Can you work these out from the model? Positions are in its coordinate system, mm. Coordinates: 2 decimals unless noted, no trailing zeros. Order: outer loops, then holes, each group sorted by start corner. A loop starts at its lowest first (then second) coordinate and runs counter-clockwise, first axis right, second up. Notation, with made-up numbers: M -29.5,-27 L 29.5,-27 A22 cw 29.5,9 Z; hole C 14,65.5 d3. An arc over 180 degrees is marked long. Answer as CSV lines item,"result". Start each with the question number.
1. I need wall thicknesses on line 1 along Y through (x, z) = (218, 2.5); line 2 along Y through (x, z) = (196.85, 1.2); line 3 along Y through (x, z) = (66.5, 3.2). Which ranges of each line are inside material? Lowest first, please. Write a range as from..to.
2. Will this pin go through, and if not, where does the flat tip stop? pin 1 (3 mm diameter, centred on x = 424, z = 3.5, fed in from +Y).
3. If we section it at A-A (x = 50.8): List the corners of the cut face in (y, z) for me, plus the area to 3 significant figures.
4. If we section it at B-B (z = 3.1): Give the number of separate pieces and of enclosed holes in the cut face, plus the area to 3 significant figures.
5. If we section it at C-C (y = 230): List the corners of the cut face in (x, z) for me, plus the area to 3 significant figures.
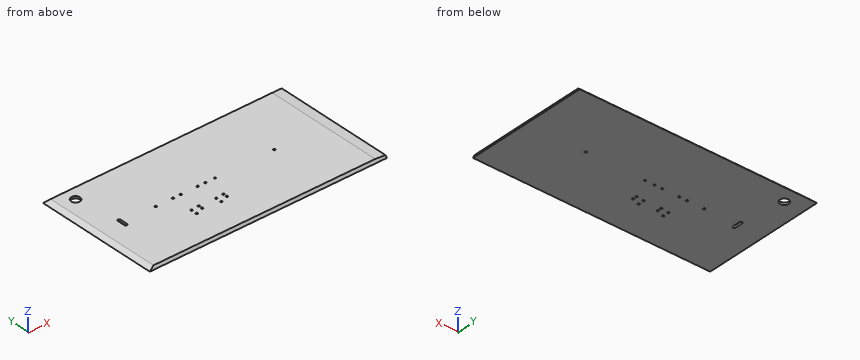
Autodesk Inventor part; units mm, degrees
ref_plane "YZ Plane" through (0, 0, 0) normal (1, 0, 0) x (0, 1, 0)
ref_plane "XY Plane" through (0, 0, 0) normal (0, 0, 1) x (1, 0, 0)
sketch "Sketch1" plane through (0, 0, 0) normal (0, 0, 1) x (1, 0, 0)
  line L0 (0, 0) -> (609.6, 0)
  line L1 (609.6, 0) -> (609.6, 317.881)
  line L2 (609.6, 317.881) -> (0, 317.881)
  line L3 (0, 317.881) -> (0, 0)
  dimension "d0" = 609.6
  dimension "d1" = 317.881
extrude "Extrusion1" add sketch "Sketch1" along normal blind 5.7658
sketch "Sketch2" plane through (0, 317.881, 0) normal (0, 1, 0) x (1, 0, 0)
  line L0 (609.6, 0) -> (0, 0)
  line L1 (0, 0) -> (0, -5.7658)
  line L2 (609.6, -5.7658) -> (0, -5.7658)
  line L3 (609.6, 0) -> (609.6, -5.7658)
  line L4 (0, 0) -> (609.6, 0)
  line L5 (0, 0) -> (14.4594, -5.7658)
  line L6 (0, -5.7658) -> (609.6, -5.7658)
  line L7 (14.4594, -5.7658) -> (14.4594, 0)
  line L8 (14.4594, -5.7658) -> (20.2252, -5.7658) construction
  dimension "d4" = 21.74
  dimension "d5" = 90
extrude "Extrusion2" cut sketch "Sketch2" against normal through all contours L5 L2 L1
sketch "Sketch3" plane through (609.6, 0, 0) normal (1, 0, 0) x (0, 0, -1)
  line L0 (0, 0) -> (0, 317.881)
  line L1 (0, 317.881) -> (-5.7658, 317.881)
  line L2 (-5.7658, 0) -> (-5.7658, 317.881)
  line L3 (0, 0) -> (-5.7658, 0)
  line L4 (0, 0) -> (-5.7658, 0)
  line L5 (0, 0) -> (-5.7658, 5.7658)
  line L6 (-5.7658, 0) -> (-5.7658, 317.881)
  line L7 (0, 0) -> (8.1541, 0) construction
  line L8 (0, 317.881) -> (-5.7658, 317.881)
  line L9 (0, 317.881) -> (-5.7658, 312.1152)
  line L10 (0, 317.881) -> (8.1541, 317.881) construction
  dimension "d8" = 135
  dimension "d9" = 135
extrude "Extrusion3" cut sketch "Sketch3" against normal through all contours L3 L2 L5 | L9 L2 L1
ref_plane "Center Plane" through (0, 158.9405, 0) normal (0, 1, 0) x (-1, 0, 0)
sketch "Sketch4" plane through (0, 158.9405, 0) normal (0, 1, 0) x (-1, 0, 0)
  line L0 (-14.4594, 5.7658) -> (0, 0)
  line L1 (-609.6, 5.7658) -> (-14.4594, 5.7658)
  line L2 (-609.6, 0) -> (-609.6, 5.7658)
  line L3 (-609.6, 0) -> (0, 0)
  line L4 (-609.6, 5.7658) -> (-584.2, 5.7658) construction
  line L5 (-584.2, 5.7658) -> (-609.6, 4.4413)
  point P0 (0, 0)
  dimension "d13" = 25.4
  dimension "d14" = 2.985
extrude "Extrusion4" cut sketch "Sketch4" against normal through all both and the other way through all contours L5 L2 L1
sketch "Sketch5" plane through (0, 0, 5.7658) normal (0, 0, 1) x (1, 0, 0)
  circle A0 centre (196.85, 158.9278) radius 2.5019
  line L0 (0, 317.881) -> (0, 0)
  line L1 (609.6, 317.881) -> (0, 317.881)
  circle A1 centre (260.35, 158.9405) radius 2.5019
  circle A2 centre (196.85, 103.5558) radius 2.5019
  circle A3 centre (260.35, 103.5685) radius 2.5019
  circle A4 centre (196.85, 88.3158) radius 2.5019
  circle A5 centre (260.35, 88.3285) radius 2.5019
  circle A6 centre (152.4, 158.9405) radius 2.5019
  circle A7 centre (304.8, 158.9405) radius 2.5019
  circle A8 centre (457.2, 158.9405) radius 2.5019
  line L2 (66.675, 145.7528) -> (67.325, 145.7528)
  line L3 (70.5, 148.9278) -> (70.5, 168.9278)
  line L4 (67.325, 172.1028) -> (66.675, 172.1028)
  line L5 (63.5, 168.9278) -> (63.5, 148.9278)
  line L6 (63.5, 145.7528) -> (70.5, 172.1028) construction
  line L7 (70.5, 145.7528) -> (63.5, 172.1028) construction
  arc A9 (70.5, 168.9278) -> (67.325, 172.1028) centre (67.325, 168.9278) ccw
  arc A10 (66.675, 172.1028) -> (63.5, 168.9278) centre (66.675, 168.9278) ccw
  arc A11 (63.5, 148.9278) -> (66.675, 145.7528) centre (66.675, 148.9278) ccw
  arc A12 (67.325, 145.7528) -> (70.5, 148.9278) centre (67.325, 148.9278) ccw
  point P0 (67, 158.9278)
  dimension "d17" = 196.85
  dimension "d18" = 158.9532
  dimension "d19" = 5.0038
  dimension "d20" = 63.5
  dimension "d21" = 5.0038
  dimension "d22" = 55.372
  dimension "d23" = 55.372
  dimension "d24" = 196.85
  dimension "d25" = 63.5
  dimension "d26" = 158.9405
  dimension "d27" = 5.0038
  dimension "d28" = 5.0038
  dimension "d29" = 15.24
  dimension "d30" = 15.24
  dimension "d31" = 5.0038
  dimension "d32" = 5.0038
  dimension "d33" = 63.5
  dimension "d34" = 196.85
  dimension "d35" = 152.4
  dimension "d36" = 5.0038
  dimension "d37" = 158.9405
  dimension "d38" = 304.8
  dimension "d39" = 5.0038
  dimension "d40" = 158.9405
  dimension "d41" = 457.2
  dimension "d42" = 158.9405
  dimension "d43" = 5.0038
  dimension "d44" = 3.175
  dimension "d45" = 7
  dimension "d46" = 20
  dimension "d47" = 158.9532
  dimension "d48" = 63.5
extrude "Extrusion5" cut sketch "Sketch5" against normal through all
sketch "Sketch6" plane through (0, 0, 5.7658) normal (0, 0, 1) x (1, 0, 0)
  circle A0 centre (50.8, 279.781) radius 11.43
  line L0 (609.6, 317.881) -> (0, 317.881)
  line L1 (0, 317.881) -> (0, 0)
  dimension "d51" = 38.1
  dimension "d52" = 50.8
  dimension "d53" = 22.86
extrude "Extrusion6" cut sketch "Sketch6" against normal through all
sketch "Sketch7" plane through (0, 0, 5.7658) normal (0, 0, 1) x (1, 0, 0)
  circle A0 centre (216.85, 158.9278) radius 2.5
  circle A1 centre (196.85, 103.5558) radius 2.5019 construction
  circle A2 centre (196.85, 158.9278) radius 2.5019 construction
  line L0 (196.85, 103.5558) -> (196.85, 158.9278) construction
  line L1 (196.85, 158.9278) -> (216.85, 158.9278) construction
  line L2 (216.85, 158.9278) -> (216.85, 105.4278) construction
  circle A3 centre (216.85, 105.4278) radius 2.5
  circle A4 centre (196.85, 88.3158) radius 2.5019 construction
  line L3 (196.85, 103.5558) -> (196.85, 88.3158) construction
  line L4 (216.85, 95.4278) -> (216.85, 105.4278) construction
  circle A5 centre (216.85, 95.4278) radius 2.5
  line L5 (216.85, 158.9278) -> (280.35, 158.9278) construction
  line L6 (280.35, 158.9278) -> (280.35, 95.4278) construction
  line L7 (280.35, 95.4278) -> (280.35, 105.4278) construction
  circle A6 centre (280.35, 105.4278) radius 2.5
  circle A7 centre (280.35, 95.4278) radius 2.5
  circle A8 centre (280.35, 158.9278) radius 2.5
  circle A9 centre (260.35, 158.9405) radius 2.5019
  point P0 (0, 0)
  dimension "d56" = 5
  dimension "d57" = 20
  dimension "d58" = 5
  dimension "d59" = 5
  dimension "d60" = 63.5
  dimension "d61" = 5
  dimension "d62" = 5
  dimension "d63" = 5
  dimension "d64" = 63.5
  dimension "d65" = 63.5
  dimension "d66" = 10
  dimension "d67" = 180
  dimension "d68" = 10
extrude "Extrusion7" cut sketch "Sketch7" against normal through all contours A0 | A3 | A5 | A6 | A7 | A8
properties part number "Wind Tunnel Test Section Bottom" material "Polycarbonate, Clear"
Solved:
1,line 1,"2.5..93.21, 97.65..103.21, 107.65..156.71, 161.15..315.38"
1,line 2,"1.2..85.81, 90.82..101.05, 106.06..156.43, 161.43..316.68"
1,line 3,"3.2..145.76, 172.1..314.68"
2,pin 1,"y = 315.88"
3,outline,"M 0,0 L 268.35,0 L 268.35,5.77 L 5.77,5.77 Z; M 291.21,0 L 317.88,0 L 312.12,5.77 L 291.21,5.77 Z"
3,area,"1,670 mm²"
4,separate pieces,"1"
4,enclosed holes,"17"
4,area,"187,000 mm²"
5,outline,"M 0,0 L 609.6,0 L 609.6,4.44 L 584.2,5.77 L 14.46,5.77 Z"
5,area,"3,460 mm²"
